from build123d import *

# Parameters (mm, degrees)
SKETCH1_W                    = 105
SKETCH1_H                    = 40
BASE_FLANGE1_DEPTH           = 3
EDGE_FLANGE1_STRIP_W         = 18
EDGE_FLANGE1_STRIP_H         = 3
EDGE_FLANGE1_STRIP_CUT_DEPTH = 40
EDGE_FLANGE1_DEPTH           = 40
F_25_0_1495_DIAMETER_SLOT1_D = 3.7973
F_3_0MM_START                = -37.361157767
F_3_0MM_DOWEL_SLOT1_DEPTH    = 3
F_3_0MM_DOWEL_SLOT2_D        = 8


# Read off the part's stored shape, not the designer's step: Ø3.0mm Dowel Slot1
# Sheet-metal steps are written as plain solids
with BuildPart() as part:
    # Sketch1 → Base-Flange1 (new body)
    with BuildSketch(Plane.XY):
        with Locations((18.138842233, 4.62628866)):
            Rectangle(SKETCH1_W, SKETCH1_H)
    extrude(amount=-BASE_FLANGE1_DEPTH)

    # Edge-Flange1 strip (across the edge) → Edge-Flange1 strip cut (cut)
    with BuildSketch(Plane(origin=(-34.361157767, 24.62628866, 0), x_dir=(1, 0, 0), z_dir=(0, -1, 0))):
        with Locations((-6, -1.5)):
            Rectangle(EDGE_FLANGE1_STRIP_W, EDGE_FLANGE1_STRIP_H)
    extrude(amount=EDGE_FLANGE1_STRIP_CUT_DEPTH, mode=Mode.SUBTRACT)

    # Edge-Flange1 section (across the edge) → Edge-Flange1 (add)
    with BuildSketch(Plane(origin=(-34.361157767, 24.62628866, 0), x_dir=(1, 0, 0), z_dir=(0, -1, 0))):
        with BuildLine():
            Line((-3, 3), (-3, 55))
            Line((-3, 55), (0, 55))
            Line((0, 55), (0, 3))
            ThreePointArc((0, 3), (0.878679656, 0.878679656), (3, 0))
            Line((3, 0), (3, -3))
            ThreePointArc((3, -3), (-1.242640687, -1.242640687), (-3, 3))
        make_face()
    extrude(amount=EDGE_FLANGE1_DEPTH)

    # #25 (0.1495) Diameter Slot1 (through all)
    with Locations(Plane(origin=(0, 0, -3), x_dir=(-1, 0, 0), z_dir=(0, 0, -1))):
        with Locations((-60.638842233, 19.62628866), (-60.638842233, -10.37371134), (21.361157767, -10.37371134), (21.361157767, 19.62628866)):
            Hole(F_25_0_1495_DIAMETER_SLOT1_D / 2)

    # Ø3.0mm Dowel Slot1 outline → Ø3.0mm Dowel Slot1 (cut)
    with BuildSketch(Plane.YZ.offset(F_3_0MM_START)):
        with BuildLine():
            Line((6.67117218, 31.008782935), (6.671169071, 31.013782934))
            ThreePointArc((6.671169071, 31.013782934), (4.920081294, 32.762694482), (3.171169747, 31.011606705))
            Line((3.171169747, 31.011606705), (3.171172856, 31.006606706))
            ThreePointArc((3.171172856, 31.006606706), (4.922260632, 29.257695159), (6.67117218, 31.008782935))
        make_face()
        with BuildLine():
            Line((-4.562452858, 9.334806586), (-4.562455966, 9.339806585))
            ThreePointArc((-4.562455966, 9.339806585), (-6.313543742, 11.088718132), (-8.06245529, 9.337630356))
            Line((-8.06245529, 9.337630356), (-8.062452181, 9.332630357))
            ThreePointArc((-8.062452181, 9.332630357), (-6.311364405, 7.583718809), (-4.562452858, 9.334806586))
        make_face()
        with BuildLine():
            Line((15.836935374, 8.38259529), (15.836932265, 8.387595289))
            ThreePointArc((15.836932265, 8.387595289), (14.085844489, 10.136506836), (12.336932941, 8.38541906))
            Line((12.336932941, 8.38541906), (12.33693605, 8.380419061))
            ThreePointArc((12.33693605, 8.380419061), (14.088023826, 6.631507514), (15.836935374, 8.38259529))
        make_face()
    extrude(amount=F_3_0MM_DOWEL_SLOT1_DEPTH, mode=Mode.SUBTRACT)

    # Ø3.0mm Dowel Slot2 (through all)
    with Locations(Plane.ZY.offset(37.361157767)):
        with Locations((8.860112823, 3.887240042)):
            Hole(F_3_0MM_DOWEL_SLOT2_D / 2)


solid = part.part
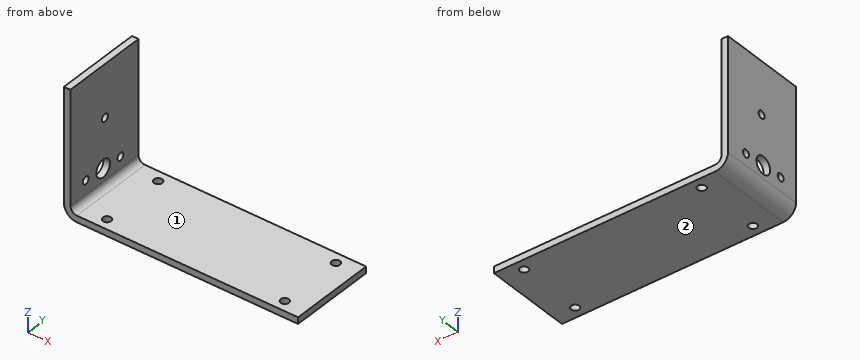
Source: CAD feature listing. Evaluate the final solid. Frame: model axes, mm. Face numbers are marked on the shaded views. A direction names the side the tool comes from. Round coordinates to 2 decimals unless told otherwise and drop trailing zeros. Loops run counter-clockwise (first coordinate to the right, second up) from the corner with the lowest first, then second, coordinate; pieces in that order, holes last. Notation, with made-up numbers: (21.5, -20.5) - (63.5, -20.5) arc R17 cw to (63.5, 8.5) - close; hole circle Ø5 at (53.25, 76). An arc over 180 degrees is marked (long way). Write item = value, one per line. Start each with the question number.
(1) Section query A-A, the plane y = 11. Output: boundary loops of the cut face in (x, z), plus the area to 3 significant figures.
(2) Section query D-D, the plane z = 51. Output: boundary loops of the cut face in (x, y), plus the area to 3 significant figures.
(3) Section query B-B, the plane y = -6. Output: boundary loops of the cut face in (x, z), plus the area to 3 significant figures.
(4) Section query C-C, the plane x = 47. Output: boundary loops of the cut face in (y, z), plus the area to 3 significant figures.
(5) Set-up query: the marked faces 1 and 2. Return all of +Z, -Z, +X, -X, +Y, -Y with unobstructed straight access to the full face (end or side cutting, diameter ignored); none if empty.
(6) Ray query, line 1 along Z through (x, y) = (-11.5, -1.5); line 2 along X through (y, z) = (-11.5, 33); line 3 along Z through (x, y) = (-32.5, -4). Return the intervals inside material, ascending. Write a range as from..to.
(7) Pin query (flat end, axial travel): pin 1 (5 mm diameter, centred on x = 60.64, y = -10.37, fed in from +Z); pin 2 (12 mm diameter, centred on y = 4, z = 28, fed in from +X). Return the tip coordinate at first contact, or that it passes through.
Conclusion:
q1.outline = (-37.36, 3) arc R6 ccw to (-31.36, -3) - (70.64, -3) - (70.64, 0) - (-31.36, 0) arc R3 cw to (-34.36, 3) - (-34.36, 55) - (-37.36, 55) - close
q1.area = 483 mm2
q2.outline = (-37.36, -15.37) - (-34.36, -15.37) - (-34.36, 24.63) - (-37.36, 24.63) - close
q2.area = 120 mm2
q3.outline = (-37.36, 3) arc R6 ccw to (-31.36, -3) - (70.64, -3) - (70.64, 0) - (-31.36, 0) arc R3 cw to (-34.36, 3) - (-34.36, 7.61) - (-37.36, 7.61) - close; (-37.36, 11.06) - (-34.36, 11.06) - (-34.36, 55) - (-37.36, 55) - close
q3.area = 473 mm2
q4.outline = (-15.37, -3) - (24.63, -3) - (24.63, 0) - (-15.37, 0) - close
q4.area = 120 mm2
q5.face_1 = +Z, +X, +Y, -Y
q5.face_2 = -Z, +X, -X, +Y, -Y
q6.line_1 = -3..0
q6.line_2 = -37.36..-34.36
q6.line_3 = -2.89..0.22
q7.pin_1 = 0
q7.pin_2 = -34.36
